from build123d import *

# Parameters (mm, degrees)
F1_DEPTH  = 45
F2_R      = 4.125
F3_DEPTH  = 10
F4_R      = 4.125
F5_DEPTH  = 10
F6_R      = 4.125
F7_DEPTH  = 20
F8_R      = 3
F10_DEPTH = 3
F11_R     = 6


with BuildPart() as f1:
    # F0 (on Top) → F1 (new body)
    with BuildSketch(Plane.XY):
        with BuildLine():
            Line((29.698485, 29.698485), (0, 0))
            Line((0, 0), (-29.698485, 29.698485))
            Line((-29.698485, 29.698485), (-36.769553, 22.627417))
            Line((-36.769553, 22.627417), (-13.80761, -0.334525))
            ThreePointArc((-13.80761, -0.334525), (-31.069176, -11.738608), (-40.792156, -30))
            ThreePointArc((-40.792156, -30), (-41.398908, -32.919715), (-41.796954, -35.875124))
            Line((-41.796954, -35.875124), (-32.248766, -32.998781))
            ThreePointArc((-32.248766, -32.998781), (33, -40), (-32.248766, -47.001219))
            Line((-32.248766, -47.001219), (-41.796954, -44.124876))
            ThreePointArc((-41.796954, -44.124876), (-41.398908, -47.080285), (-40.792156, -50))
            ThreePointArc((-40.792156, -50), (28.261392, -71.069176), (13.80761, -0.334525))
            Line((13.80761, -0.334525), (36.769553, 22.627417))
            Line((36.769553, 22.627417), (29.698485, 29.698485))
        make_face()
        with BuildLine():
            ThreePointArc((-41.796954, -35.875124), (-41.398908, -32.919715), (-40.792156, -30))
            Line((-40.792156, -30), (-55.973206, -30))
            Line((-55.973206, -30), (-55.973206, -38.5))
            Line((-55.973206, -38.5), (-41.973206, -38.5))
            ThreePointArc((-41.973206, -38.5), (-41.905637, -37.186182), (-41.796954, -35.875124))
        make_face()
        with BuildLine():
            Line((-55.973206, -50), (-40.792156, -50))
            ThreePointArc((-40.792156, -50), (-41.398908, -47.080285), (-41.796954, -44.124876))
            ThreePointArc((-41.796954, -44.124876), (-41.905637, -42.813818), (-41.973206, -41.5))
            Line((-41.973206, -41.5), (-55.973206, -41.5))
            Line((-55.973206, -41.5), (-55.973206, -50))
        make_face()
    extrude(amount=F1_DEPTH)

    # F2 (on face) → F3 (cut, through all)
    with BuildSketch(Plane(origin=(0, 0, 0), x_dir=(-0.707107, -0.707107, 0), z_dir=(-0.707107, 0.707107, 0))):
        with Locations((-25.4, 15)):
            Circle(F2_R)
    extrude(amount=-F3_DEPTH, mode=Mode.SUBTRACT)

    # F4 (on face) → F5 (cut, through all)
    with BuildSketch(Plane(origin=(0, 0, 0), x_dir=(-0.707107, 0.707107, 0), z_dir=(0.707107, 0.707107, 0))):
        with Locations((25.4, 15)):
            Circle(F4_R)
    extrude(amount=-F5_DEPTH, mode=Mode.SUBTRACT)

    # F6 (on face) → F7 (cut, through all)
    with BuildSketch(Plane.XZ.offset(50)):
        with Locations((-48.382681, 33.75)):
            Circle(F6_R)
        with Locations((-48.382681, 11.25)):
            Circle(F6_R)
    extrude(amount=-F7_DEPTH, mode=Mode.SUBTRACT)

    # F8
    f8_edges = [f1.edges().sort_by_distance(p)[0] for p in [
        (-55.973206, -34.25, 45),
        (-55.973206, -45.75, 45),
        (-55.973206, -45.75, 0),
        (-55.973206, -34.25, 0),
        (-33.234019, 26.162951, 45),
        (33.234019, 26.162951, 45),
        (33.234019, 26.162951, 0),
        (-33.234019, 26.162951, 0),
        (-40.792156, -30, 22.5),
        (-40.792156, -50, 22.5),
    ]]
    fillet(f8_edges, radius=F8_R)

    # F9 (on face) → F10 (cut)
    with BuildSketch(Plane(origin=(0, -30, 0), x_dir=(-1, 0, 0), z_dir=(0, 1, 0))):
        Polygon((55.307681, 37.748151), (48.382681, 41.746301), (41.457681, 37.748151), (41.457681, 29.751849), (48.382681, 25.753699), (55.307681, 29.751849), align=None)
        Polygon((55.307681, 7.251849), (55.307681, 15.248151), (48.382681, 19.246301), (41.457681, 15.248151), (41.457681, 7.251849), (48.382681, 3.253699), align=None)
    extrude(amount=-F10_DEPTH, mode=Mode.SUBTRACT)

    # F11
    f11_edges = [f1.edges().sort_by_distance(p)[0] for p in [
        (-13.80761, -0.334525, 22.5),
        (13.80761, -0.334525, 22.5),
    ]]
    fillet(f11_edges, radius=F11_R)


solid = f1.part
Source: CAD feature listing. Evaluate the final solid. Frame: model axes, mm. A direction names the side the tool comes from. Round coordinates to 2 decimals unless told otherwise and drop trailing zeros. Loops run counter-clockwise (first coordinate to the right, second up) from the corner with the lowest first, then second, coordinate; pieces in that order, holes last. Notation, with made-up numbers: (70.5, 70) - (96.5, 70) arc R29 ccw to (96.5, 105) - close; hole circle Ø3 at (-3.75, 47). An arc over 180 degrees is marked (long way). Write item = value, one per line. Start each with the question number.
(1) Set-up query: faces 1 (the face through (-49, -30, 22)), 2 (the face through (-51.797, -31.479, 5.225)), 3 (the face through (-41.907, -37.205, 22.185)). Return all of +Z, -Z, +X, -X, +Y, -Y with unobstructed straight access to the full face (end or side cutting, diameter ignored); none if empty.
(2) Section query A-A, the plane x = 7.5. Output: boundary loops of the cut face in (y, z), plus the area to 3 significant figures.
(3) Section query B-B, the plane z = 33.75. State how many separate pieces and enclosed holes the cut face has, plus the area to 3 significant figures.
(4) Ray query, line 1 along Y through (x, z) = (-44.5, 4); line 2 along Y through (x, z) = (28, 2); line 3 along X through (y, z) = (-18.5, 13). Return the intervals inside material, ascending. Write a range as from..to.
(5) Pull-direction query (X, two-part tool) for faces 4 (the face through (-18.165, 0.799, 22.815)), 5 (the face through (-44.87, -31.48, 27.78)), 6 (the face through (-49, -41.5, 22)); classes: +X half, -X half, draft (parallel to the pull), parting line (faces both ways), or undercut.
(6) Pin query (flat end, axial travel): pin 1 (12 mm diameter, centred on y = 4, z = 38.5, fed in from -X); pin 2 (3 mm diameter, centred on x = -19, z = 39.5, fed in from -Y); pin 3 (0.8 mm diameter, centred on x = -42.5, z = 35.5, fed in from -Y). Return the tip coordinate at first contact, or that it passes through.
(7) Section query C-C, the plane z = 40.5. Output: boundary loops of the cut face in (x, y), plus the area to 3 significant figures.
Conclusion:
q1.face_1 = +Z, -Z, -X, +Y
q1.face_2 = +Y
q1.face_3 = +Z, -Z
q2.outline = (-81.32, 0) - (-72.14, 0) - (-72.14, 45) - (-81.32, 45) - close; (-7.86, 0) - (7.5, 0) - (7.5, 45) - (-7.86, 45) - close
q2.area = 1,100 mm2
q3.separate_pieces = 3
q3.enclosed_holes = 0
q3.area = 2,850 mm2
q4.line_1 = -50..-41.5, -38.5..-30
q4.line_2 = -71.3..-57.46, -22.54..-8.7, 13.86..28
q4.line_3 = -36.08..-25.03, 25.03..36.08
q5.face_4 = -X half
q5.face_5 = undercut
q5.face_6 = draft
q6.pin_1 = -24.14
q6.pin_2 = -78.18
q6.pin_3 = -50.17
q7.outline = (-55.97, -50) - (-43.08, -50) arc R3 cw to (-40.21, -52.13) arc R42 ccw (long way) to (21.11, -3.69) arc R6 cw to (19.88, 5.74) - (36.77, 22.63) - (29.7, 29.7) - (0, 0) - (-29.7, 29.7) - (-36.77, 22.63) - (-19.88, 5.74) arc R6 cw to (-21.11, -3.69) arc R42 ccw to (-40.21, -27.87) arc R3 cw to (-43.08, -30) - (-46.22, -30) - (-46.22, -33) - (-50.54, -33) - (-50.54, -30) - (-55.97, -30) - (-55.97, -38.5) - (-41.97, -38.5) arc R42 cw to (-41.8, -35.88) - (-32.25, -33) arc R33 cw (long way) to (-32.25, -47) - (-41.8, -44.12) arc R42 cw to (-41.97, -41.5) - (-55.97, -41.5) - close
q7.area = 2,990 mm2
